```python
from build123d import *

# Parameters (mm, degrees)
SKETCH1_R           = 12.5
BOSS_EXTRUDE1_DEPTH = 7.5
CUT_EXTRUDE1_REACH  = 25.184
SKETCH8_W           = 12.25
SKETCH8_H           = 12.25
CUT_EXTRUDE4_REACH  = 25.184
SKETCH11_R          = 1.45


with BuildPart() as part:
    # Sketch1 → Boss-Extrude1 (new, symmetric)
    with BuildSketch(Plane.XY):
        Circle(SKETCH1_R)
    extrude(amount=BOSS_EXTRUDE1_DEPTH, both=True)

    # Sketch8 → Cut-Extrude1 (cut, up to next)
    with BuildSketch(Plane.XY.offset(7.5), mode=Mode.PRIVATE) as cut_extrude1_sk1:
        Rectangle(SKETCH8_W, SKETCH8_H)
    cut_extrude1_tool1 = extrude(cut_extrude1_sk1.sketch, amount=-CUT_EXTRUDE1_REACH, mode=Mode.PRIVATE) & part.part
    add(cut_extrude1_tool1.solids().sort_by_distance((0, 0, 7.5))[0], mode=Mode.SUBTRACT)

    # Sketch11 → Cut-Extrude4 (cut, up to next)
    with BuildSketch(Plane.XY.offset(7.5), mode=Mode.PRIVATE) as cut_extrude4_sk1:
        with Locations((7.5, 0)):
            Circle(SKETCH11_R)
    cut_extrude4_tool1 = extrude(cut_extrude4_sk1.sketch, amount=-CUT_EXTRUDE4_REACH, mode=Mode.PRIVATE) & part.part
    # Sketch11 → Cut-Extrude4 (cut, up to next)
    with BuildSketch(Plane.XY.offset(7.5), mode=Mode.PRIVATE) as cut_extrude4_sk2:
        with Locations((0, -7.5)):
            Circle(SKETCH11_R)
    cut_extrude4_tool2 = extrude(cut_extrude4_sk2.sketch, amount=-CUT_EXTRUDE4_REACH, mode=Mode.PRIVATE) & part.part
    # Sketch11 → Cut-Extrude4 (cut, up to next)
    with BuildSketch(Plane.XY.offset(7.5), mode=Mode.PRIVATE) as cut_extrude4_sk3:
        with Locations((-7.5, 0)):
            Circle(SKETCH11_R)
    cut_extrude4_tool3 = extrude(cut_extrude4_sk3.sketch, amount=-CUT_EXTRUDE4_REACH, mode=Mode.PRIVATE) & part.part
    # Sketch11 → Cut-Extrude4 (cut, up to next)
    with BuildSketch(Plane.XY.offset(7.5), mode=Mode.PRIVATE) as cut_extrude4_sk4:
        with Locations((0, 7.5)):
            Circle(SKETCH11_R)
    cut_extrude4_tool4 = extrude(cut_extrude4_sk4.sketch, amount=-CUT_EXTRUDE4_REACH, mode=Mode.PRIVATE) & part.part
    add(cut_extrude4_tool1.solids().sort_by_distance((7.5, 0, 7.5))[0], mode=Mode.SUBTRACT)
    add(cut_extrude4_tool2.solids().sort_by_distance((0, -7.5, 7.5))[0], mode=Mode.SUBTRACT)
    add(cut_extrude4_tool3.solids().sort_by_distance((-7.5, 0, 7.5))[0], mode=Mode.SUBTRACT)
    add(cut_extrude4_tool4.solids().sort_by_distance((0, 7.5, 7.5))[0], mode=Mode.SUBTRACT)


solid = part.part
```
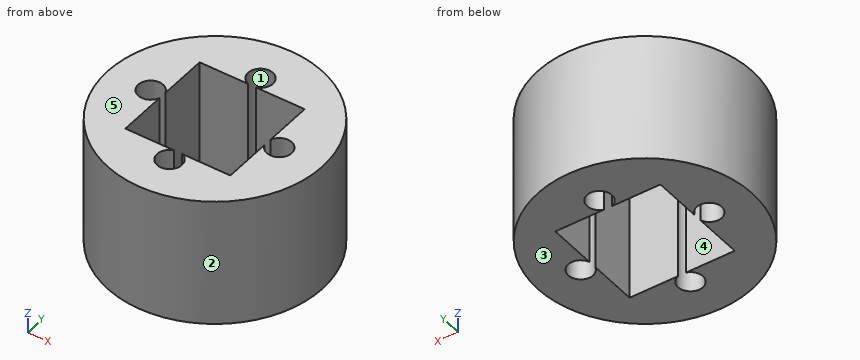
The model under review builds one solid part; all positions refer to its coordinate system, in mm. Face numbers are marked on the shaded views. A direction names the side the tool comes from. Round coordinates to 2 decimals unless told otherwise and drop trailing zeros. Loops run counter-clockwise (first coordinate to the right, second up) from the corner with the lowest first, then second, coordinate; pieces in that order, holes last.
1) Wall thickness on line 1 along Y through (x, z) = (0, 2.5); line 2 along Y through (x, z) = (-8.75, -0.75); line 3 along X through (y, z) = (-2, -3.5) (3 decimals): over which ranges is each line inside the solid? List them lowest first.
Values follow:
line 1: y = -12.5 to -8.95, 8.95 to 12.5
line 2: y = -8.93 to -0.73, 0.73 to 8.93
line 3: x = -12.339 to -6.125, 6.125 to 12.339
2) Clearance check with flat-ended pins moving along their axes: P1, Ø8, axis at x = -3, z = 1, coming from the -Y side; P2, Ø8, axis at x = -8.5, z = -4, coming from the +Y side; P3, Ø1.7, axis at x = -4, z = 3, coming from the -Y side; P4, Ø3, axis at x = -4, z = 0, coming from the +Y side. State where each tip first meets the part, or that it passes through.
Values follow:
P1: stops at y = -12.5
P2: stops at y = 11.66
P3: stops at y = -12.1
P4: stops at y = 12.25
3) Consider section C-C on z = -2.25. State the section outline as (x, y) points (3 decimals), then the cut area to 3 significant figures.
Values follow:
outline: circle Ø25 at (0, 0); hole (-6.125, -6.125) - (-0.46, -6.125) arc R1.45 ccw (long way) to (0.46, -6.125) - (6.125, -6.125) - (6.125, -0.46) arc R1.45 ccw (long way) to (6.125, 0.46) - (6.125, 6.125) - (0.46, 6.125) arc R1.45 ccw (long way) to (-0.46, 6.125) - (-6.125, 6.125) - (-6.125, 0.46) arc R1.45 ccw (long way) to (-6.125, -0.46) - close
area: 315 mm2
4) The part is to be moulded in two halves that separate along Y. For the marked faces 1, 2 and 3, say which applies: pulls with the +Y half, pulls with the -Y half, needs draft (parallel to the pull), parting line crosses it, or undercut.
Values follow:
face 1: undercut
face 2: parting line crosses it
face 3: needs draft
5) Consider section A-A on x = -7.5. State the section outline as (y, z) points, then the cut area to 4 significant figures.
Values follow:
outline: (-10, -7.5) - (-1.45, -7.5) - (-1.45, 7.5) - (-10, 7.5) - close; (1.45, -7.5) - (10, -7.5) - (10, 7.5) - (1.45, 7.5) - close
area: 256.5 mm2
6) Tool access review of the marked faces 4 and 5: name each direction out of +Z, -Z, +X, -X, +Y, -Y from which nothing blocks a thin tool from reaching the whole face with its end or side.
Values follow:
face 4: +Z, -Z
face 5: +Z, +X, -X, +Y, -Y
7) Consider section D-D on y = 10. State the section outline as (x, z) points, then the cut area to 3 significant figures.
Values follow:
outline: (-7.5, -7.5) - (7.5, -7.5) - (7.5, 7.5) - (-7.5, 7.5) - close
area: 225 mm2
